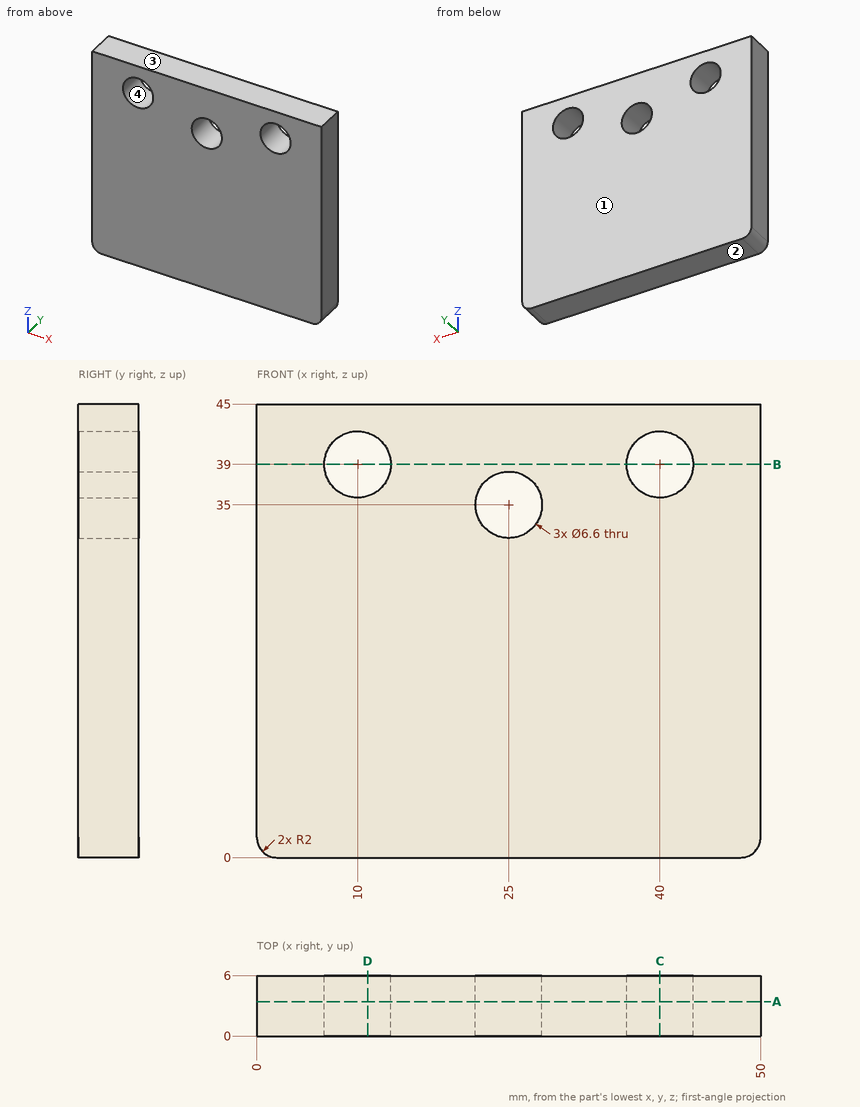
Can you work these out from the drawing? Everything is in mm from the part's minimum corner. Coordinates: 2 decimals unless noted, no trailing zeros. Write each loop counter-clockwise with the first axis right and the second up, starting at its lowest first coordinate (ties: lowest second). Pieces come first, ordered by that corner, then holes. Notation, with made-up numbers: (27, 64.5) - (67, 64.5) arc R13 ccw to (67, 73.5) - close; hole circle Ø10 at (30, -16.5). An arc over 180 degrees is marked (long way). One line per item, written item: value.
1) We'd pull the mould along Z, two halves only. Please class the marked faces 1, 2, 3 and 4: pulls with the +Z half, pulls with the -Z half, needs draft (parallel to the pull), parting line crosses it, or undercut.
Model answer:
face 1: needs draft
face 2: pulls with the -Z half
face 3: pulls with the +Z half
face 4: undercut
2) I'm going to push a flat-ended pin straight in: P1, Ø5.5, axis at x = 25, z = 35, coming from the +Y side. Where does the tip first touch, or does it pass through?
Model answer:
P1: passes through
3) Suppose I cut it at D-D on x = 11. Write out the boundary of the cut face in (y, z), and give its area (3 significant figures).
Model answer:
outline: (0, 0) - (6, 0) - (6, 35.86) - (0, 35.86) - close; (0, 42.14) - (6, 42.14) - (6, 45) - (0, 45) - close
area: 232 mm²
4) Suppose I cut it at C-C on x = 40. Write out the boundary of the cut face in (y, z).
Model answer:
outline: (0, 0) - (6, 0) - (6, 35.7) - (0, 35.7) - close; (0, 42.3) - (6, 42.3) - (6, 45) - (0, 45) - close
5) Suppose I cut it at A-A on y = 3.4. Write out the boundary of the cut face in (x, z).
Model answer:
outline: (0, 2) arc R2 ccw to (2, 0) - (48, 0) arc R2 ccw to (50, 2) - (50, 45) - (0, 45) - close; hole circle Ø6.6 at (10, 39); hole circle Ø6.6 at (25, 35); hole circle Ø6.6 at (40, 39)
6) Suppose I cut it at B-B on z = 39. Write out the boundary of the cut face in (x, y).
Model answer:
outline: (0, 0) - (6.7, 0) - (6.7, 6) - (0, 6) - close; (13.3, 0) - (36.7, 0) - (36.7, 6) - (13.3, 6) - close; (43.3, 0) - (50, 0) - (50, 6) - (43.3, 6) - close
7) I need wall thicknesses on line 1 along Z through (x, y) = (10, 3.45); line 2 along X through (y, z) = (0.9, 34.5); line 3 along X through (y, z) = (5, 34). Which ranges of each line are inside material? Lowest first, please.
Model answer:
line 1: z = 0 to 35.7, 42.3 to 45
line 2: x = 0 to 21.74, 28.26 to 50
line 3: x = 0 to 21.86, 28.14 to 50
